Here's how the part is built. I have some questions about the finished solid (model axes, mm). Face numbers are marked on the shaded views. A direction names the side the tool comes from. Round coordinates to 2 decimals unless told otherwise and drop trailing zeros. Write each loop counter-clockwise with the first axis right and the second up, starting at its lowest first coordinate (ties: lowest second). Pieces come first, ordered by that corner, then holes. Notation, with made-up numbers: M 69.25,8 L 99.25,8 A9 cw 99.25,24 Z; hole C 3,-14.75 d5. An arc over 180 degrees is marked long. Use one line per item in the form item = value. Start each with the question number.
Q1. I need wall thicknesses on line 1 along Z through (x, y) = (81, 0); line 2 along Z through (x, y) = (-44.5, -1.75); line 3 along Y through (x, z) = (-40.5, 1.5). Which ranges of each line are inside material? Lowest first, please. Write a range as from..to.
Q2. I want a section at A-A on y = -6. List the corners of the cut face in (x, z) for me, and give its area (3 significant figures).
Q3. For the marked faces 1, 2 and 3, which set-ups out of +Z, -Z, +X, -X, +Y, -Y let a thin tool reach every point of the face, with its end or its side?
Q4. I want a section at D-D on x = -54. List the corners of the cut face in (y, z) for me, and give its area (3 significant figures).
Q5. I want a section at C-C on x = 29. List the corners of the cut face in (y, z) for me (1 decimal).
Q6. I'm going to push flat-ended pins straight in: pin 1 Ø1.5 at (x, y) = (39, -6) entering from -Z; pin 2 Ø2.5 at (x, z) = (-12, 1) entering from +Y; pin 3 Ø4 at (x, z) = (54.5, 2) entering from -Y. Where does each tip first touch, or does it pass through?
Q7. I want a section at B-B on z = 7.25. List the corners of the cut face in (x, y) for me.
```python
from build123d import *

# Parameters (mm, degrees)
SKETCH1_R               = 14.2875
BOSS_EXTRUDE1_DEPTH     = 31.75
CUT_EXTRUDE1_DEPTH      = 63.5
SKETCH3_R               = 12.7
BOSS_EXTRUDE2_DEPTH     = 76.2
SKETCH4_R               = 12.7
BOSS_EXTRUDE3_DEPTH     = 76.2
SKETCH5_R               = 1.5875
CUT_EXTRUDE2_DEPTH      = 6.35
CIRPATTERN1_COUNT       = 4
MIRROR1_COPY_1_SKETCH_R = 1.5875
MIRROR1_COPY_1_DEPTH    = 6.35
MIRROR1_COPY_2_SKETCH_R = 1.5875
MIRROR1_COPY_2_DEPTH    = 6.35
MIRROR1_COPY_3_SKETCH_R = 1.5875
MIRROR1_COPY_3_DEPTH    = 6.35


with BuildPart() as part:
    # Sketch1 → Boss-Extrude1 (new body, symmetric)
    with BuildSketch(Plane(origin=(0, 0, 0), x_dir=(0, 0, -1), z_dir=(1, 0, 0))):
        Circle(SKETCH1_R)
    extrude(amount=BOSS_EXTRUDE1_DEPTH, both=True)

    # Sketch2 → Cut-Extrude1 (cut)
    with BuildSketch(Plane(origin=(31.75, 0, 0), x_dir=(0, 0, -1), z_dir=(1, 0, 0))):
        with BuildLine():
            Line((0, 11.90625), (2.38125, 11.90625))
            Line((2.38125, 11.90625), (2.38125, 14.087664984))
            ThreePointArc((2.38125, 14.087664984), (0, 14.2875), (-2.38125, 14.087664984))
            Line((-2.38125, 14.087664984), (-2.38125, 11.90625))
            Line((-2.38125, 11.90625), (0, 11.90625))
        make_face()
    extrude(amount=-CUT_EXTRUDE1_DEPTH, mode=Mode.SUBTRACT)

    # Sketch3 → Boss-Extrude2 (add)
    with BuildSketch(Plane(origin=(31.75, 0, 0), x_dir=(0, 0, -1), z_dir=(1, 0, 0))):
        with Locations(Location((0, 0, 0), (0, 0, 100.806922875))):  # turned: the seam where the file's is
            Circle(SKETCH3_R)
    extrude(amount=BOSS_EXTRUDE2_DEPTH)

    # Sketch4 → Boss-Extrude3 (add)
    with BuildSketch(Plane.ZY.offset(31.75)):
        with Locations(Location((0, 0, 0), (0, 0, 79.193077125))):  # turned: the seam where the file's is
            Circle(SKETCH4_R)
    extrude(amount=BOSS_EXTRUDE3_DEPTH)

    # Sketch5 → Cut-Extrude2 (cut)
    with BuildSketch(Plane(origin=(107.95, 0, 0), x_dir=(0, 0, -1), z_dir=(1, 0, 0))):
        with Locations((0, 12.7)):
            Circle(SKETCH5_R)
    cut_extrude2 = extrude(amount=-CUT_EXTRUDE2_DEPTH, mode=Mode.SUBTRACT)

    # CirPattern1: Cut-Extrude2 ×4 about axis
    cirpattern1_axis = Axis((0, 0, 0), (1, 0, 0))
    for i in range(1, CIRPATTERN1_COUNT):
        add(cut_extrude2.rotate(cirpattern1_axis, i * 360 / CIRPATTERN1_COUNT), mode=Mode.SUBTRACT)

    # Mirror1: Cut-Extrude2 across plane
    add(cut_extrude2.mirror(Plane(origin=(0, 0, 0), x_dir=(0, 0, 1), z_dir=(1, 0, 0))), mode=Mode.SUBTRACT)

    # Mirror1 copy 1 sketch → Mirror1 copy 1 (cut)
    with BuildSketch(Plane(origin=(-107.95, 0, 0), x_dir=(0, 1, 0), z_dir=(-1, 0, 0))):
        with Locations((0, -12.7)):
            Circle(MIRROR1_COPY_1_SKETCH_R)
    extrude(amount=-MIRROR1_COPY_1_DEPTH, mode=Mode.SUBTRACT)

    # Mirror1 copy 2 sketch → Mirror1 copy 2 (cut)
    with BuildSketch(Plane.ZY.offset(107.95)):
        with Locations((0, -12.7)):
            Circle(MIRROR1_COPY_2_SKETCH_R)
    extrude(amount=-MIRROR1_COPY_2_DEPTH, mode=Mode.SUBTRACT)

    # Mirror1 copy 3 sketch → Mirror1 copy 3 (cut)
    with BuildSketch(Plane(origin=(-107.95, 0, 0), x_dir=(0, -1, 0), z_dir=(-1, 0, 0))):
        with Locations((0, -12.7)):
            Circle(MIRROR1_COPY_3_SKETCH_R)
    extrude(amount=-MIRROR1_COPY_3_DEPTH, mode=Mode.SUBTRACT)


solid = part.part
```
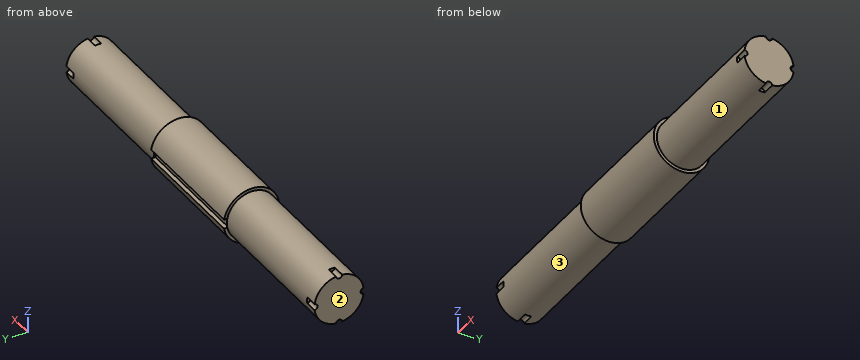
Reported:
q1.line_1 = -12.7..12.7
q1.line_2 = -12.58..12.58
q1.line_3 = -12.61..12.61
q2.outline = M -107.95,-11.19 L -31.75,-11.19 L -31.75,-12.97 L 31.75,-12.97 L 31.75,-11.19 L 107.95,-11.19 L 107.95,11.19 L 31.75,11.19 L 31.75,12.97 L -31.75,12.97 L -31.75,11.19 L -107.95,11.19 Z
q2.area = 5,060 mm^2
q3.face_1 = +X
q3.face_2 = +Z, -Z, -X, +Y, -Y
q3.face_3 = -X
q4.outline = C 0,0 d25.4
q4.area = 507 mm^2
q5.outline = M 11.9,-2.4 L 11.9,2.4 L 14.1,2.4 A14.3 ccw long 14.1,-2.4 Z
q6.pin_1 = -11.56
q6.pin_2 = 11.91
q6.pin_3 = -12.7
q7.outline = M -107.95,-10.43 L -31.75,-10.43 L -31.75,-12.31 L 31.75,-12.31 L 31.75,-10.43 L 107.95,-10.43 L 107.95,10.43 L 31.75,10.43 L 31.75,12.31 L -31.75,12.31 L -31.75,10.43 L -107.95,10.43 Z
